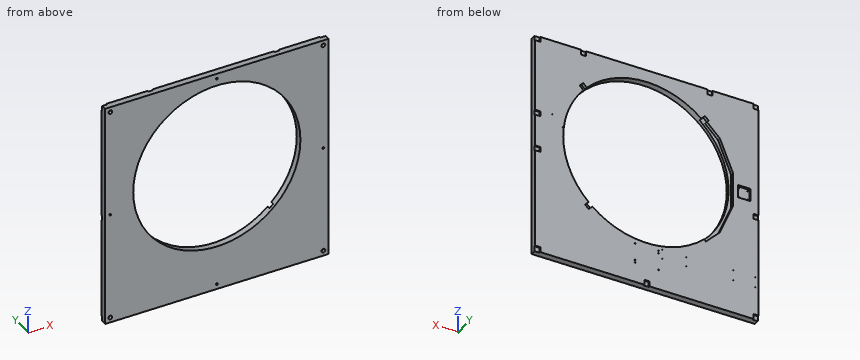
from build123d import *

# Parameters (mm, degrees)
SKETCH1_W             = 2000
SKETCH1_H             = 2000
BOSS_EXTRUDE1_DEPTH   = 50
SKETCH2_R             = 6
CUT_EXTRUDE1_DEPTH    = 30
SKETCH3_W             = 2000
SKETCH3_H             = 50
CUT_EXTRUDE2_DEPTH    = 250
SKETCH4_W             = 1750
SKETCH4_H             = 50
CUT_EXTRUDE3_DEPTH    = 125
SKETCH5_W             = 1750
SKETCH5_H             = 50
CUT_EXTRUDE4_DEPTH    = 125
SKETCH6_R             = 655
CUT_EXTRUDE5_DEPTH    = 51
SKETCH7_W             = 100
SKETCH7_H             = 100
CUT_EXTRUDE6_DEPTH    = 15
M8_TAPPED_HOLE1_D     = 6.8
M8_TAPPED_HOLE1_DEPTH = 17.707073895
M8_TAPPED_HOLE1_TIP   = 2.042926105
SKETCH13_R            = 15
SKETCH13_R_2          = 7.5
CUT_EXTRUDE8_DEPTH    = 25
SKETCH14_W            = 40
SKETCH14_H            = 40
SKETCH14_W_2          = 80
SKETCH14_H_2          = 80
CUT_EXTRUDE9_DEPTH    = 10
M5_TAPPED_HOLE1_D     = 4.2
M5_TAPPED_HOLE1_DEPTH = 12.4
M5_TAPPED_HOLE1_TIP   = 1.2618073
M8_TAPPED_HOLE2_D     = 6.8
M8_TAPPED_HOLE2_DEPTH = 19.75
M8_TAPPED_HOLE2_TIP   = 2.042926105
SKETCH21_R            = 4
CUT_EXTRUDE10_DEPTH   = 10
M6_TAPPED_HOLE1_D     = 5
M6_TAPPED_HOLE1_DEPTH = 15
M6_TAPPED_HOLE1_TIP   = 1.502151548
CUT_EXTRUDE11_DEPTH   = 25
CUT_EXTRUDE12_DEPTH   = 25


with BuildPart() as part:
    # Sketch1 → Boss-Extrude1 (new body)
    with BuildSketch(Plane(origin=(0, 0, 0), x_dir=(1, 0, 0), z_dir=(0, 1, 0))):
        Rectangle(SKETCH1_W, SKETCH1_H)
    extrude(amount=-BOSS_EXTRUDE1_DEPTH)

    # Sketch2 → Cut-Extrude1 (cut)
    with BuildSketch(Plane(origin=(0, 0, 0), x_dir=(1, 0, 0), z_dir=(0, 1, 0))):
        with Locations((0, -175)):
            Circle(SKETCH2_R)
        with Locations((106, 129)):
            Circle(SKETCH2_R)
    extrude(amount=-CUT_EXTRUDE1_DEPTH, mode=Mode.SUBTRACT)

    # Sketch3 → Cut-Extrude2 (cut)
    with BuildSketch(Plane.XY.offset(1000)):
        with Locations((0, -25)):
            Rectangle(SKETCH3_W, SKETCH3_H)
    extrude(amount=-CUT_EXTRUDE2_DEPTH, mode=Mode.SUBTRACT)

    # Sketch4 → Cut-Extrude3 (cut)
    with BuildSketch(Plane.ZY.offset(1000)):
        with Locations((-125, -25)):
            Rectangle(SKETCH4_W, SKETCH4_H)
    extrude(amount=-CUT_EXTRUDE3_DEPTH, mode=Mode.SUBTRACT)

    # Sketch5 → Cut-Extrude4 (cut)
    with BuildSketch(Plane(origin=(1000, 0, 0), x_dir=(0, 0, -1), z_dir=(1, 0, 0))):
        with Locations((125, -25)):
            Rectangle(SKETCH5_W, SKETCH5_H)
    extrude(amount=-CUT_EXTRUDE4_DEPTH, mode=Mode.SUBTRACT)

    # Sketch6 → Cut-Extrude5 (cut, through all)
    with BuildSketch(Plane(origin=(0, 0, 0), x_dir=(1, 0, 0), z_dir=(0, 1, 0))):
        Circle(SKETCH6_R)
    extrude(amount=-CUT_EXTRUDE5_DEPTH, mode=Mode.SUBTRACT)

    # Sketch7 → Cut-Extrude6 (cut)
    with BuildSketch(Plane(origin=(0, 0, 0), x_dir=(1, 0, 0), z_dir=(0, 1, 0))):
        with Locations((-763, 0)):
            Rectangle(SKETCH7_W, SKETCH7_H)
    extrude(amount=-CUT_EXTRUDE6_DEPTH, mode=Mode.SUBTRACT)

    # M8 Tapped Hole1
    with Locations(Plane(origin=(0, -15, 0), x_dir=(1, 0, 0), z_dir=(0, 1, 0))):
        with Locations((-798, 35), (-798, -35), (-728, -35), (-728, 35)):
            Hole(M8_TAPPED_HOLE1_D / 2, depth=M8_TAPPED_HOLE1_DEPTH)
            with Locations((0, 0, -(M8_TAPPED_HOLE1_DEPTH + M8_TAPPED_HOLE1_TIP / 2))):  # 118° drill point
                Cone(0, M8_TAPPED_HOLE1_D / 2, M8_TAPPED_HOLE1_TIP, mode=Mode.SUBTRACT)

    # Sketch13 → Cut-Extrude8 (cut)
    with BuildSketch(Plane.XZ.offset(50)):
        with Locations((-835, 710)):
            Circle(SKETCH13_R)
        with Locations((835, -960)):
            Circle(SKETCH13_R)
        with Locations((835, 710)):
            Circle(SKETCH13_R)
        with Locations((-835, -960)):
            Circle(SKETCH13_R)
        with Locations((0, -960)):
            Circle(SKETCH13_R_2)
        with Locations((0, 710)):
            Circle(SKETCH13_R_2)
        with Locations((835, -125)):
            Circle(SKETCH13_R_2)
        with Locations((-835, -125)):
            Circle(SKETCH13_R_2)
    extrude(amount=-CUT_EXTRUDE8_DEPTH, mode=Mode.SUBTRACT)

    # Sketch14 → Cut-Extrude9 (cut)
    with BuildSketch(Plane(origin=(0, 0, 0), x_dir=(1, 0, 0), z_dir=(0, 1, 0))):
        with Locations((855, -730)):
            Rectangle(SKETCH14_W, SKETCH14_H)
        with Locations((875, 165)):
            Rectangle(SKETCH14_W_2, SKETCH14_H)
        with Locations((855, 980)):
            Rectangle(SKETCH14_W, SKETCH14_H)
        with Locations((-855, 980)):
            Rectangle(SKETCH14_W, SKETCH14_H)
        with Locations((-855, -730)):
            Rectangle(SKETCH14_W, SKETCH14_H)
        with Locations((-875, 165)):
            Rectangle(SKETCH14_W_2, SKETCH14_H)
        with Locations((0, 1000)):
            Rectangle(SKETCH14_W, SKETCH14_H_2)
        with Locations((-495, -750)):
            Rectangle(SKETCH14_W, SKETCH14_H_2)
        with Locations((495, -750)):
            Rectangle(SKETCH14_W, SKETCH14_H_2)
        with Locations((875, -125)):
            Rectangle(SKETCH14_W_2, SKETCH14_H)
    extrude(amount=-CUT_EXTRUDE9_DEPTH, mode=Mode.SUBTRACT)

    # M5 Tapped Hole1
    with Locations(Plane(origin=(0, 0, 0), x_dir=(1, 0, 0), z_dir=(0, 1, 0))):
        with Locations((740, -152), (740, -72), (660, -72), (660, -152), (-310.091163632, 744.682016608), (-310.091163632, 669.682016608), (-120.091163632, 669.682016608), (-120.091163632, 744.682016608)):
            Hole(M5_TAPPED_HOLE1_D / 2, depth=M5_TAPPED_HOLE1_DEPTH)
            with Locations((0, 0, -(M5_TAPPED_HOLE1_DEPTH + M5_TAPPED_HOLE1_TIP / 2))):  # 118° drill point
                Cone(0, M5_TAPPED_HOLE1_D / 2, M5_TAPPED_HOLE1_TIP, mode=Mode.SUBTRACT)

    # M8 Tapped Hole2
    with Locations(Plane(origin=(0, 0, 0), x_dir=(1, 0, 0), z_dir=(0, 1, 0))):
        with Locations((-92.500000018, 687.499999989), (92.500000005, 687.499999992), (92.500000005, 842.499999992), (-92.499999995, 842.499999992)):
            Hole(M8_TAPPED_HOLE2_D / 2, depth=M8_TAPPED_HOLE2_DEPTH)
            with Locations((0, 0, -(M8_TAPPED_HOLE2_DEPTH + M8_TAPPED_HOLE2_TIP / 2))):  # 118° drill point
                Cone(0, M8_TAPPED_HOLE2_D / 2, M8_TAPPED_HOLE2_TIP, mode=Mode.SUBTRACT)

    # Sketch21 → Cut-Extrude10 (cut)
    with BuildSketch(Plane(origin=(0, 0, 0), x_dir=(1, 0, 0), z_dir=(0, 1, 0))):
        with Locations((-92.500000018, 707.499999987)):
            Circle(SKETCH21_R)
        with Locations((92.500000005, 822.499999992)):
            Circle(SKETCH21_R)
    extrude(amount=-CUT_EXTRUDE10_DEPTH, mode=Mode.SUBTRACT)

    # M6 Tapped Hole1
    with Locations(Plane(origin=(0, 0, 0), x_dir=(1, 0, 0), z_dir=(0, 1, 0))):
        with Locations((-678.5, 738), (-678.5, 656.604373077), (-848.5, 658), (-848.5, 738)):
            Hole(M6_TAPPED_HOLE1_D / 2, depth=M6_TAPPED_HOLE1_DEPTH)
            with Locations((0, 0, -(M6_TAPPED_HOLE1_DEPTH + M6_TAPPED_HOLE1_TIP / 2))):  # 118° drill point
                Cone(0, M6_TAPPED_HOLE1_D / 2, M6_TAPPED_HOLE1_TIP, mode=Mode.SUBTRACT)

    # Sketch25 → Cut-Extrude11 (cut)
    with BuildSketch(Plane(origin=(0, 0, 0), x_dir=(1, 0, 0), z_dir=(0, 1, 0))):
        with BuildLine():
            Line((-555.28218759, -371.027695765), (-456.083873865, -470.226009489))
            Line((-456.083873865, -470.226009489), (-425.26997323, -439.412108854))
            ThreePointArc((-425.26997323, -439.412108854), (-611.483880806, 5.001505042), (-418.025396439, 446.309667686))
            Line((-418.025396439, 446.309667686), (-449.012806053, 477.297077301))
            Line((-449.012806053, 477.297077301), (-555.28218759, 371.027695765))
            Line((-555.28218759, 371.027695765), (-655, 130.287600634))
            Line((-655, 130.287600634), (-655, -130.287600634))
            Line((-655, -130.287600634), (-555.28218759, -371.027695765))
        make_face()
        Polygon((-675, -134.265847981), (-572.23736889, -382.356785712), (-470.226009489, -484.368145113), (-456.083873865, -470.226009489), (-555.28218759, -371.027695765), (-655, -130.287600634), (-655, 130.287600634), (-555.28218759, 371.027695765), (-449.012806053, 477.297077301), (-463.154941677, 491.439212925), (-572.23736889, 382.356785712), (-675, 134.265847981), align=None)
    extrude(amount=-CUT_EXTRUDE11_DEPTH, mode=Mode.SUBTRACT)

    # Sketch26 → Cut-Extrude12 (cut)
    with BuildSketch(Plane(origin=(0, 0, 0), x_dir=(1, 0, 0), z_dir=(0, 1, 0))):
        Polygon((-484.368145113, -498.510280737), (-456.083873865, -470.226009489), (-420.576835046, -491.287513165), (-456.083873865, -526.794551984), align=None)
        Polygon((526.794551984, -456.083873865), (491.287513165, -420.576835046), (470.226009489, -456.083873865), (498.510280737, -484.368145113), align=None)
        Polygon((456.083873865, 526.794551984), (420.576835046, 491.287513165), (456.083873865, 470.226009489), (484.368145113, 498.510280737), align=None)
    extrude(amount=-CUT_EXTRUDE12_DEPTH, mode=Mode.SUBTRACT)


solid = part.part
Verification items for the finished model (mm, model axes). Round coordinates to 2 decimals unless told otherwise and drop trailing zeros. Loops run counter-clockwise (first coordinate to the right, second up) from the corner with the lowest first, then second, coordinate; pieces in that order, holes last. Notation, with made-up numbers: (89, 14) - (113, 14) arc R27 ccw to (113, 36) - close; hole circle Ø5 at (4.5, -32). An arc over 180 degrees is marked (long way). Answer in a Markdown table with one row per item. Add a question column.
Q1. Section check A-A on z = 0. Enter the section's corners in (x, y), plus the area to 3 significant figures.
Q2. Section check C-C on z = -266. Enter the section's corners in (x, y).
Q3. Material ranges on line 1 (X direction, y = -6, z = -658); line 2 (Z direction, x = -798, y = -27); line 3 (X direction, y = -32, z = 710), recorded low to high.
Q4. Section check D-D on x = 628.5. Enter the section's corners in (y, z), plus the area to 3 significant figures.
Q5. Gauge pin test, flat ends, axial feed: pin 1 (8 mm diameter, centred on y = -2.5, z = -988, fed in from -X); pin 2 (11 mm diameter, centred on y = -3.5, z = 728, fed in from +X); pin 3 (11 mm diameter, centred on x = 862, y = -3, fed in from -Z). Record the tip position at first contact, or that the pin passes through.
Q6. Section check B-B on x = 131. Enter the section's corners in (y, z).
Found:
| question | item | result |
|---|---|---|
| 1 | outline | (-875, -50) - (-655, -50) - (-655, -25) - (-675, -25) - (-675, 0) - (-713, 0) - (-713, -15) - (-813, -15) - (-813, 0) - (-875, 0) - close; (655, -50) - (875, -50) - (875, 0) - (655, 0) - close |
| 1 | area | 20,000 mm² |
| 2 | outline | (-875, -50) - (-598.56, -50) - (-598.56, -25) - (-620.43, -25) - (-620.43, 0) - (-875, 0) - close; (598.56, -50) - (875, -50) - (875, 0) - (598.56, 0) - close |
| 3 | line 1 | x = -875 to -851, -846 to -680.57, -676.43 to 875 |
| 3 | line 2 | z = -1000 to -38.4, -31.6 to 31.6, 38.4 to 750 |
| 3 | line 3 | x = -875 to -850, -820 to -7.5, 7.5 to 820, 850 to 875 |
| 4 | outline | (-50, -1000) - (0, -1000) - (0, -184.43) - (-50, -184.43) - close; (-50, 184.43) - (0, 184.43) - (0, 750) - (-50, 750) - close |
| 4 | area | 69,100 mm² |
| 5 | pin 1 | stops at x = -835 |
| 5 | pin 2 | stops at x = 835 |
| 5 | pin 3 | stops at z = -960 |
| 6 | outline | (-50, -1000) - (0, -1000) - (0, -641.77) - (-50, -641.77) - close; (-50, 641.77) - (0, 641.77) - (0, 750) - (-50, 750) - close |
